Design review of the part built by this model. Coordinates are the model's own, in mm. Coordinates: 2 decimals unless noted, no trailing zeros. Write each loop counter-clockwise with the first axis right and the second up, starting at its lowest first coordinate (ties: lowest second). Pieces come first, ordered by that corner, then holes. Notation, with made-up numbers: (-18, -2.75) - (30, -2.75) arc R35 cw to (30, 29.25) - close; hole circle Ø9 at (64, 1.25). An arc over 180 degrees is marked (long way). One line per item, written item: value.
from build123d import *

# Parameters (mm, degrees)
F1_DEPTH = 18.5674


with BuildPart() as f1:
    # F0 (on Top) → F1 (new body)
    with BuildSketch(Plane.XY):
        Polygon((7.728108, -22.929351), (19.729705, -14.007767), (24.195226, 0.264309), (19.418992, 14.435427), (7.225363, 23.092703), (-7.728108, 22.929351), (-19.729705, 14.007767), (-24.195226, -0.264309), (-19.418992, -14.435427), (-7.225363, -23.092703), align=None)
    extrude(amount=-F1_DEPTH)


solid = f1.part
1. Consider section C-C, the plane y = -12. Write out the cut boundary in (x, z), then the cut area to 3 significant figures.
Answer block:
outline: (-20.24, -18.57) - (20.36, -18.57) - (20.36, 0) - (-20.24, 0) - close
area: 754 mm^2
2. Consider section B-B, the plane x = -16.5. Write out the cut boundary in (y, z).
Answer block:
outline: (-16.51, -18.57) - (16.41, -18.57) - (16.41, 0) - (-16.51, 0) - close
3. Consider section A-A, the plane z = -14.75. Write out the cut boundary in (x, y), then the cut area to 3 significant figures.
Answer block:
outline: (-24.2, -0.26) - (-19.42, -14.44) - (-7.23, -23.09) - (7.73, -22.93) - (19.73, -14.01) - (24.2, 0.26) - (19.42, 14.44) - (7.23, 23.09) - (-7.73, 22.93) - (-19.73, 14.01) - close
area: 1,720 mm^2
4. Insertion check: pin 1 Ø1 at (y, z) = (-3, -10) entering from +X; pin 2 Ø3 at (x, z) = (12, -2.5) entering from -Y; pin 3 Ø1.5 at (y, z) = (-16, -12) entering from +X. Each pin has a flat end and moves straight along its axis. Give the tip position at first contact, or say it passes through.
Answer block:
pin 1: stops at x = 23.33
pin 2: stops at y = -20.87
pin 3: stops at x = 18.06
5. Wall thickness on line 1 along Y through (x, z) = (-18, -3.25); line 2 along X through (y, z) = (1, -7.25); line 3 along Y through (x, z) = (16, -9): over which ranges is each line inside the solid? List them lowest first.
Answer block:
line 1: y = -15.44 to 15.29
line 2: x = -23.8 to 23.95
line 3: y = -16.78 to 16.86
